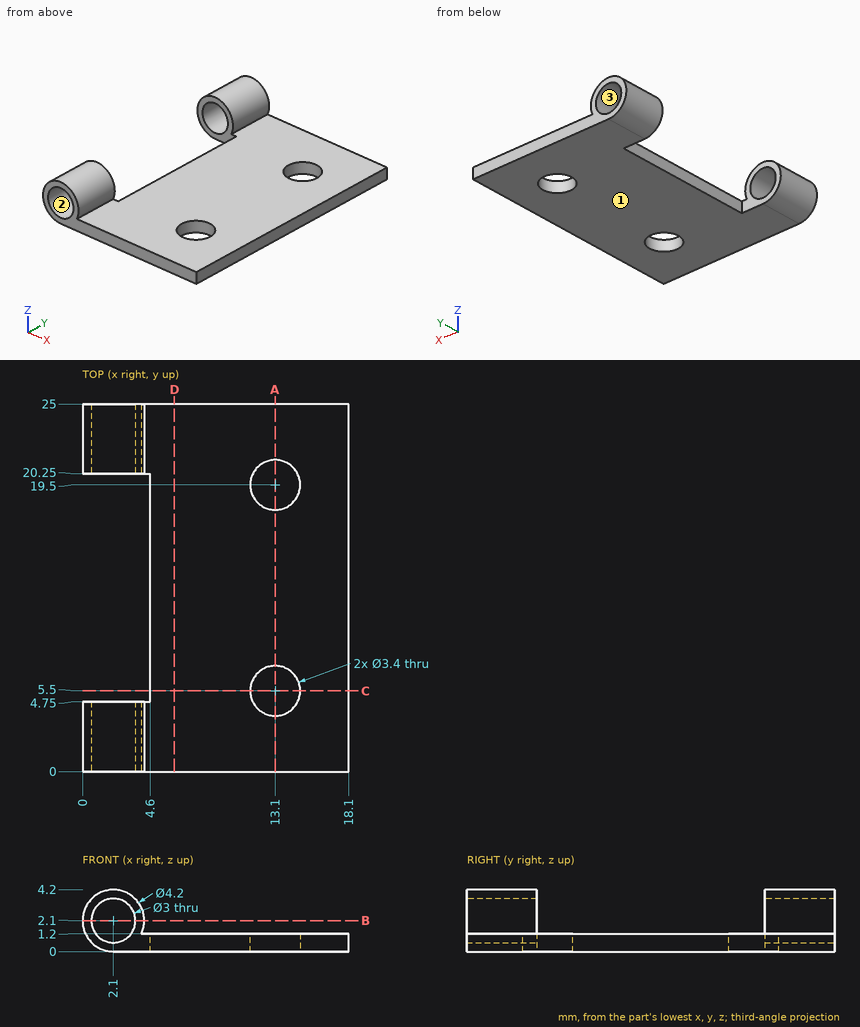
Study the drawing (mm; zero at the part's minimum x, y, z) and answer. Give positions to 0.01 mm unless a question says otherwise; leave off trailing zeros. Order: outer loops, then holes, each group sorted by start corner. A loop starts at its lowest first (then second) coordinate and runs counter-clockwise, first axis right, second up. Notation, with made-up numbers: (62.5, -3.75) - (88.5, -3.75) arc R23 ccw to (88.5, 22.25) - close; hole circle Ø7 at (30.5, 83). An arc over 180 degrees is marked (long way). Answer in a Markdown table with one row per item. Add a question column.
Q1. The part is cut by section B-B (z = 2.1). Determine the outline of the cut face in (x, y), then the cut area to 3 significant figures.
Q2. The part is cut by section A-A (x = 13.1). Determine the outline of the cut face in (y, z), then the cut area to 3 significant figures.
Q3. Given P1, Ø5.5, axis at x = 13.1, y = 5.5, coming from the +Z side; P2, Ø1.3, axis at y = 12.5, z = 1, coming from the -X side, each flat-ended and moving along its own axis, determine where each tip first touches the part or whether it passes through.
Q4. Find the intervals of material crossed by line 1 along Y through (x, z) = (13.1, 0.3); line 2 along X through (y, z) = (2.9, 2.1); line 3 along Y through (x, z) = (1.5, 3.9), in increasing order. Write a range as [from, to].
Q5. The part is cut by section C-C (y = 5.5). Determine the outline of the cut face in (x, z).
Q6. The part is cut by section D-D (x = 6.25). Determine the outline of the cut face in (y, z), then the cut area to 3 significant figures.
Q7. For a pull along X with two mould halves and no side action, classify the marked faces 1, 2 and 3 as released by +X, released by -X, zero draft, split by the parting line, or undercut.
Determined:
| question | item | result |
|---|---|---|
| 1 | outline | (0, 0) - (0.6, 0) - (0.6, 4.75) - (0, 4.75) - close; (0, 20.25) - (0.6, 20.25) - (0.6, 25) - (0, 25) - close; (3.6, 0) - (4.2, 0) - (4.2, 4.75) - (3.6, 4.75) - close; (3.6, 20.25) - (4.2, 20.25) - (4.2, 25) - (3.6, 25) - close |
| 1 | area | 11.4 mm² |
| 2 | outline | (0, 0) - (3.8, 0) - (3.8, 1.2) - (0, 1.2) - close; (7.2, 0) - (17.8, 0) - (17.8, 1.2) - (7.2, 1.2) - close; (21.2, 0) - (25, 0) - (25, 1.2) - (21.2, 1.2) - close |
| 2 | area | 21.8 mm² |
| 3 | P1 | stops at z = 1.2 |
| 3 | P2 | stops at x = 4.6 |
| 4 | line 1 | y = [0, 3.8], [7.2, 17.8], [21.2, 25] |
| 4 | line 2 | x = [0, 0.6], [3.6, 4.2] |
| 4 | line 3 | y = [0, 4.75], [20.25, 25] |
| 5 | outline | (4.6, 0) - (11.4, 0) - (11.4, 1.2) - (4.6, 1.2) - close; (14.8, 0) - (18.1, 0) - (18.1, 1.2) - (14.8, 1.2) - close |
| 6 | outline | (0, 0) - (25, 0) - (25, 1.2) - (0, 1.2) - close |
| 6 | area | 30.0 mm² |
| 7 | face 1 | zero draft |
| 7 | face 2 | undercut |
| 7 | face 3 | undercut |
